Work out the finished part from the listing and answer in its coordinate system (mm). Coordinates: 2 decimals unless noted, no trailing zeros. Loops run counter-clockwise (first coordinate to the right, second up) from the corner with the lowest first, then second, coordinate; pieces in that order, holes last. Notation, with made-up numbers: (68.25, -14) -> (91.25, -14) arc R24 ccw to (91.25, 7) -> close; hole circle Ø7 at (66.25, -13.5). An arc over 180 degrees is marked (long way). Answer as CSV lines item,"result".
Autodesk Inventor part; units mm, degrees
ref_plane "YZ Plane" through (0, 0, 0) normal (1, 0, 0) x (0, 1, 0)
ref_plane "XZ Plane" through (0, 0, 0) normal (0, 1, 0) x (-1, 0, 0)
ref_plane "XY Plane" through (0, 0, 0) normal (0, 0, 1) x (1, 0, 0)
sketch "Sketch1" plane through (0, 0, 0) normal (0, 1, 0) x (-1, 0, 0)
  line L0 (14.35, -100) -> (-14.35, -100)
  line L1 (14.35, 0) -> (14.35, -100)
  line L2 (14.35, 0) -> (-14.35, 0)
  line L3 (14.35, 0) -> (-14.35, 0)
  line L4 (-14.35, -100) -> (-14.35, 0)
  point P0 (0, 0)
extrude "Extrusion1" add sketch "Sketch1" along normal blind 5
sketch "Sketch2" plane through (0, 5, 0) normal (0, 1, 0) x (1, 0, 0)
  circle A0 centre (0, 80) radius 2.5
  circle A1 centre (0, 90) radius 2.5
  circle A2 centre (0, 10) radius 2.5
  point P0 (0, 0)
extrude "Extrusion2" cut sketch "Sketch2" against normal through all
properties part number "plat"
(1) A cutting plane is placed at D-D, the plane z = -78.5. Write down the section's boundary in (x, y), and give its area (4 significant figures).
Computed values:
outline,"(-14.35, 0) -> (-2, 0) -> (-2, 5) -> (-14.35, 5) -> close; (2, 0) -> (14.35, 0) -> (14.35, 5) -> (2, 5) -> close"
area,"123.5 mm2"
(2) A cutting plane is placed at B-B, the plane y = 2.25. Write down the section's boundary in (x, z), and give its area (3 significant figures).
Computed values:
outline,"(-14.35, -100) -> (14.35, -100) -> (14.35, 0) -> (-14.35, 0) -> close; hole circle Ø5 at (0, -90); hole circle Ø5 at (0, -80); hole circle Ø5 at (0, -10)"
area,"2,810 mm2"
(3) Consider line 1 along Z through (x, y) = (0, 2.1); line 2 along X through (y, z) = (3.2, -90); line 3 along Z through (x, y) = (-2.25, 3.15). Determine where each line is inside the solid, lowest interval first.
Computed values:
line 1,"-100 to -92.5, -87.5 to -82.5, -77.5 to -12.5, -7.5 to 0"
line 2,"-14.35 to -2.5, 2.5 to 14.35"
line 3,"-100 to -91.09, -88.91 to -81.09, -78.91 to -11.09, -8.91 to 0"
(4) A cutting plane is placed at C-C, the plane x = 0.5. Write down the section's boundary in (y, z).
Computed values:
outline,"(0, -100) -> (5, -100) -> (5, -92.45) -> (0, -92.45) -> close; (0, -87.55) -> (5, -87.55) -> (5, -82.45) -> (0, -82.45) -> close; (0, -77.55) -> (5, -77.55) -> (5, -12.45) -> (0, -12.45) -> close; (0, -7.55) -> (5, -7.55) -> (5, 0) -> (0, 0) -> close"
(5) For a pull along X with two mould halves and no side action, classify faces 1 (the face through (-14.35, 2, -49)), 2 (the face through (-0.54, 2.54, -7.56)), 3 (the face through (0, 0, -49)) as pulls with the +X half, pulls with the -X half, needs draft (parallel to the pull), parting line crosses it, or undercut.
Computed values:
face 1,"pulls with the -X half"
face 2,"undercut"
face 3,"needs draft"
(6) A cutting plane is placed at A-A, the plane z = -90. Write down the section's boundary in (x, y).
Computed values:
outline,"(-14.35, 0) -> (-2.5, 0) -> (-2.5, 5) -> (-14.35, 5) -> close; (2.5, 0) -> (14.35, 0) -> (14.35, 5) -> (2.5, 5) -> close"
